```python
from build123d import *

# Parameters (mm, degrees)
SALIENTE_EXTRUIR1_DEPTH = 116
SALIENTE_EXTRUIR3_DEPTH = 47.28


with BuildPart() as part:
    # Croquis1 → Saliente-Extruir1 (new body)
    with BuildSketch(Plane(origin=(0, 0, 0), x_dir=(1, 0, 0), z_dir=(0, 1, 0))):
        Polygon((-3.632503467, -6.369321148), (3.699742186, -6.330500856), (7.332245653, 0.038820292), (3.632503467, 6.369321148), (-3.699742186, 6.330500856), (-7.332245653, -0.038820292), align=None)
    extrude(amount=SALIENTE_EXTRUIR1_DEPTH)

    # Croquis6 → Saliente-Extruir3 (add)
    with BuildSketch(Plane.XZ):
        Polygon((7.332245653, -0.038820292), (3.699742186, 6.330500856), (-3.632503467, 6.369321148), (-7.332245653, 0.038820292), (-3.699742186, -6.330500856), (3.632503467, -6.369321148), align=None)
    extrude(amount=SALIENTE_EXTRUIR3_DEPTH)


solid = part.part
```
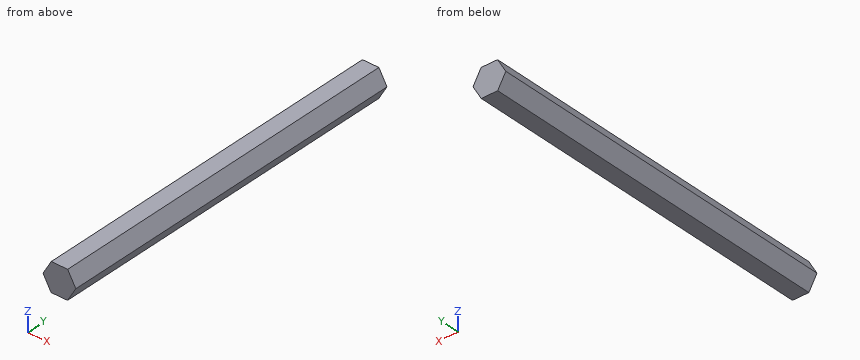
Design review of the part built by this model. Coordinates are the model's own, in mm. Coordinates: 2 decimals unless noted, no trailing zeros. Order: outer loops, then holes, each group sorted by start corner. A loop starts at its lowest first (then second) coordinate and runs counter-clockwise, first axis right, second up. Notation, with made-up numbers: M 47,38.5 L 64,38.5 A16 ccw 64,60.5 Z; hole C 75,61 d4. An arc over 180 degrees is marked long. Answer as a JSON object with one key per item and string values. Group by question number.
1) For pin 1 (5 mm diameter, centred on y = 16, z = -2.5, fed in from -X), flat-tipped, find the tip position at first contact; note if it passes through.
2) Wall thickness on L1, parallel to Z at x = -2, y = 43.5; L2, parallel to X at y = -28, z = -1.75; L3, parallel to Z at x = 1.5, y = 5: over which ranges is each line inside the solid? List them lowest first.
3) Add section C-C, the plane x = 5.75. Write out the cut boundary in (y, z).
4) Add section A-A, the plane y = 32.5. Write out the cut boundary in (x, z).
5) Add section B-B, the plane z = -2.25. Write out the cut boundary in (x, y), then the cut area to 3 significant figures.
Computed values:
{
 "1": {"pin 1": "stops at x = -7.31"},
 "2": {"L1": "z = -6.34 to 6.36", "L2": "x = -6.31 to 6.33", "L3": "z = -6.36 to 6.34"},
 "3": {"outline": "M -47.28,-2.75 L 116,-2.75 L 116,2.74 L -47.28,2.74 Z"},
 "4": {"outline": "M -7.33,0.04 L -3.7,-6.33 L 3.63,-6.37 L 7.33,-0.04 L 3.7,6.33 L -3.63,6.37 Z"},
 "5": {"outline": "M -6.03,-47.28 L 6.04,-47.28 L 6.04,116 L -6.03,116 Z", "area": "1,970 mm^2"}
}
